The listing builds one solid part. Answer for the finished solid, in the listing's coordinates (mm). A direction names the side the tool comes from. Give positions to 0.01 mm unless a question says otherwise; leave off trailing zeros. Write each loop counter-clockwise with the first axis right and the second up, starting at its lowest first coordinate (ties: lowest second). Pieces come first, ordered by that corner, then holes. Notation, with made-up numbers: (-27.5, 64.25) - (-20.5, 64.25) arc R22 cw to (-20.5, 91.25) - close; hole circle Ø10 at (-11.5, 15). An arc over 180 degrees is marked (long way). Return JSON: item names as keys, results as strings.
from build123d import *

# Parameters (mm, degrees)
SKETCH1_W           = 20
SKETCH1_H           = 30
BOSS_EXTRUDE1_DEPTH = 20
SKETCH4_W           = 12
SKETCH4_H           = 10
CUT_EXTRUDE2_DEPTH  = 18
SKETCH3_R           = 1.5
CUT_EXTRUDE3_DEPTH  = 38.416573868
SKETCH5_R           = 1.5
CUT_EXTRUDE4_DEPTH  = 10


with BuildPart() as part:
    # Sketch1 → Boss-Extrude1 (new body)
    with BuildSketch(Plane(origin=(0, 0, 0), x_dir=(1, 0, 0), z_dir=(0, 1, 0))):
        with Locations((0, 15)):
            Rectangle(SKETCH1_W, SKETCH1_H)
    extrude(amount=BOSS_EXTRUDE1_DEPTH)

    # Sketch4 → Cut-Extrude2 (cut)
    with BuildSketch(Plane(origin=(0, 20, 0), x_dir=(1, 0, 0), z_dir=(0, 1, 0))):
        with Locations((0, 20)):
            Rectangle(SKETCH4_W, SKETCH4_H)
    extrude(amount=-CUT_EXTRUDE2_DEPTH, mode=Mode.SUBTRACT)

    # Sketch3 → Cut-Extrude3 (cut, through all)
    with BuildSketch(Plane(origin=(0, 0, 0), x_dir=(1, 0, 0), z_dir=(0, 1, 0))):
        with Locations(Location((0, 20, 0), (0, 0, 270))):
            Circle(SKETCH3_R)
    extrude(amount=CUT_EXTRUDE3_DEPTH, mode=Mode.SUBTRACT)

    # Sketch5 → Cut-Extrude4 (cut)
    with BuildSketch(Plane.XY):
        with Locations((0, 15)):
            Circle(SKETCH5_R)
        with Locations(Location((0, 5, 0), (0, 0, 180))):
            Circle(SKETCH5_R)
    extrude(amount=-CUT_EXTRUDE4_DEPTH, mode=Mode.SUBTRACT)


solid = part.part
Item 1: A flat-ended cylindrical pin translates along its axis: P1, Ø0.9, axis at x = -0.5, y = 4.5, coming from the +Z side. Find the tip coordinate at first contact, or state that the pin passes through.
Answer below:
{"P1": "stops at z = -10"}
Item 2: For faces 1 (the face through (-10, 10, -15)), 2 (the face through (6, 11, -20)), 3 (the face through (0, 5, -10)), determine the directions among +Z, -Z, +X, -X, +Y, -Y from which every point of the face is accessible in a straight line to the end or side of a thin tool.
Answer below:
{"face 1": "+Z, -Z, -X, +Y, -Y", "face 2": "+Y", "face 3": "+Z"}
Item 3: A cutting plane is placed at D-D on x = 3. Determine the outline of the cut face in (y, z).
Answer below:
{"outline": "(0, -30) - (20, -30) - (20, -25) - (2, -25) - (2, -15) - (20, -15) - (20, 0) - (0, 0) - close"}
Item 4: The mould has two halves that part along X. Classify faces 4 (the face through (0, 15, -10)), 5 (the face through (0, 0, -15)), 6 (the face through (10, 10, -15)): +X half, -X half, draft (parallel to the pull), parting line (faces both ways), or undercut.
Answer below:
{"face 4": "undercut", "face 5": "draft", "face 6": "+X half"}
Item 5: A cutting plane is placed at C-C on y = 15. Determine the outline of the cut face in (x, z), then the cut area to 3 significant figures.
Answer below:
{"outline": "(-10, -30) - (10, -30) - (10, 0) - (1.5, 0) - (1.5, -10) - (-1.5, -10) - (-1.5, 0) - (-10, 0) - close; hole (-6, -25) - (6, -25) - (6, -15) - (-6, -15) - close", "area": "450 mm²"}
Item 6: Consider L1, parallel to Y at x = 0, z = -4.5; L2, parallel to Z at x = 0, y = 15.25; L3, parallel to X at y = 5, z = -2.5. Determine where each line is inside the solid, lowest interval first.
Answer below:
{"L1": "y = 0 to 3.5, 6.5 to 13.5, 16.5 to 20", "L2": "z = -30 to -25, -15 to -10", "L3": "x = -10 to -1.5, 1.5 to 10"}
Item 7: A cutting plane is placed at B-B on x = 0. Determine the outline of the cut face in (y, z), then the cut area to 3 significant figures.
Answer below:
{"outline": "(0, -30) - (20, -30) - (20, -25) - (2, -25) - (2, -21.5) - (0, -21.5) - close; (0, -18.5) - (2, -18.5) - (2, -15) - (20, -15) - (20, 0) - (16.5, 0) - (16.5, -10) - (13.5, -10) - (13.5, 0) - (6.5, 0) - (6.5, -10) - (3.5, -10) - (3.5, 0) - (0, 0) - close", "area": "354 mm²"}
Item 8: A cutting plane is placed at A-A on z = -20. Determine the outline of the cut face in (x, y), then the cut area to 3 significant figures.
Answer below:
{"outline": "(-10, 0) - (-1.5, 0) - (-1.5, 2) - (-6, 2) - (-6, 20) - (-10, 20) - close; (1.5, 0) - (10, 0) - (10, 20) - (6, 20) - (6, 2) - (1.5, 2) - close", "area": "178 mm²"}
